Autodesk Inventor part; units mm, degrees
ref_plane "YZ Plane" through (0, 0, 0) normal (1, 0, 0) x (0, 1, 0)
ref_plane "XZ Plane" through (0, 0, 0) normal (0, 1, 0) x (-1, 0, 0)
ref_plane "XY Plane" through (0, 0, 0) normal (0, 0, 1) x (1, 0, 0)
sketch "Sketch1" plane through (0, 0, 0) normal (0, 0, 1) x (1, 0, 0)
  line L0 (-40.7788, 51.9292) -> (79.2212, 51.9292)
  line L1 (79.2212, 51.9292) -> (79.2212, -68.0708)
  line L2 (79.2212, -68.0708) -> (-40.7788, -68.0708)
  line L3 (-40.7788, -68.0708) -> (-40.7788, 51.9292)
  circle A0 centre (19.2212, -8.0708) radius 19.05
  point P0 (0, 0)
  dimension "d0" = 120
  dimension "d1" = 120
  dimension "d2" = 38.1
extrude "Extrusion1" add sketch "Sketch1" along normal blind 12.7
sketch "Sketch2" plane through (0, 0, 12.7) normal (0, 0, 1) x (1, 0, 0)
  line L0 (-40.7788, 51.9292) -> (-40.7788, -68.0708)
  line L1 (-40.7788, -8.0708) -> (79.2212, -8.0708)
  line L2 (79.2212, -68.0708) -> (79.2212, 51.9292)
  line L3 (79.2212, 51.9292) -> (-40.7788, 51.9292)
  line L4 (19.2212, 51.9292) -> (19.2212, -68.0708)
  line L5 (-40.7788, -68.0708) -> (79.2212, -68.0708)
  point P0 (0, 0)
  point P1 (-25.2788, 36.4292)
  point P2 (63.7212, 36.4292)
  point P3 (63.7212, -52.5708)
  point P4 (-25.2788, -52.5708)
  dimension "d5" = 89
  dimension "d6" = 89
  dimension "d7" = 89
  dimension "d8" = 89
hole "Hole1" at (-25.2788, 36.4292, 12.7) at (63.7212, 36.4292, 12.7) at (63.7212, -52.5708, 12.7) at (-25.2788, -52.5708, 12.7) direction (0, 0, -1) diameter 10 end through all
properties part number "placa inferior"
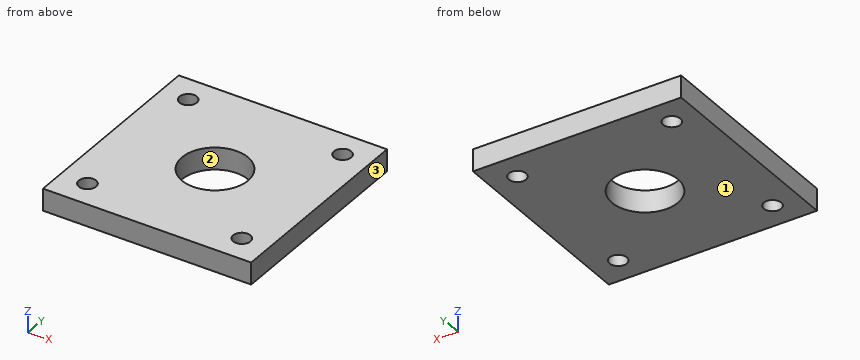
Model file for the job. Use its own axes, mm. Face numbers are marked on the shaded views. Coordinates: 2 decimals unless noted, no trailing zeros. Write each loop counter-clockwise with the first axis right and the second up, starting at its lowest first coordinate (ties: lowest second). Pieces come first, ordered by that corner, then holes. Notation, with made-up numbers: (-7, 16) - (24, 16) arc R28 cw to (24, 53) - close; hole circle Ø1 at (22, -3). An arc over 180 degrees is marked (long way). One line per question, with ' | ' between items. Start each with the question number.
Q1. Cut at A-A, the plane x = 12.5. List the corners of the cut face in (y, z), then the cut area to 3 significant figures.
Q2. Cut at B-B, the plane y = -16.5. List the corners of the cut face in (x, z).
Q3. Drill centre lines: line 1 (Y direction, x = -23, z = 3.5); line 2 (X direction, y = 33.5, z = 6.25); line 3 (X direction, y = -56, z = 3.75). Where is each one in solid material? Low to high. Write a range as [from, to].
Q4. Pin check, flat tip, straight feed: pin 1 (6 mm diameter, centred on x = 63.72, y = -52.57, fed in from +Z). Stop position of the tip, or through.
Q5. Pull direction X, two halves, no side cores. Call the marked faces 1, 2 and 3: pulls with the +X half, pulls with the -X half, needs draft (parallel to the pull), parting line crosses it, or undercut.
Q6. Cut at C-C, the plane z = 1.5. List the corners of the cut face in (x, y), then the cut area to 3 significant figures.
Answer below:
1) outline: (-68.07, 0) - (-25.9, 0) - (-25.9, 12.7) - (-68.07, 12.7) - close; (9.75, 0) - (51.93, 0) - (51.93, 12.7) - (9.75, 12.7) - close | area: 1,070 mm^2
2) outline: (-40.78, 0) - (2.14, 0) - (2.14, 12.7) - (-40.78, 12.7) - close; (36.3, 0) - (79.22, 0) - (79.22, 12.7) - (36.3, 12.7) - close
3) line 1: [-68.07, -57.02], [-48.12, 31.98], [40.88, 51.93] | line 2: [-40.78, -29.33], [-21.23, 59.67], [67.77, 79.22] | line 3: [-40.78, -28.92], [-21.64, 60.08], [67.36, 79.22]
4) pin 1: through
5) face 1: needs draft | face 2: undercut | face 3: pulls with the +X half
6) outline: (-40.78, -68.07) - (79.22, -68.07) - (79.22, 51.93) - (-40.78, 51.93) - close; hole circle Ø10 at (-25.28, -52.57); hole circle Ø10 at (-25.28, 36.43); hole circle Ø38.1 at (19.22, -8.07); hole circle Ø10 at (63.72, -52.57); hole circle Ø10 at (63.72, 36.43) | area: 12,900 mm^2
